```python
from build123d import *

# Parameters (mm, degrees)
F0_W     = 80
F0_H     = 36
F0_W_2   = 74
F0_H_2   = 25
F1_DEPTH = 1.6
F2_DEPTH = 8.5
F3_D     = 2.5
F4_R     = 1


with BuildPart() as f1:
    # F0 (on Top) → F1 (new body)
    with BuildSketch(Plane.XY):
        Rectangle(F0_W, F0_H)
        Rectangle(F0_W_2, F0_H_2, mode=Mode.SUBTRACT)
        Rectangle(F0_W_2, F0_H_2)
    extrude(amount=-F1_DEPTH)

    # F0 (on Top) → F2 (join)
    with BuildSketch(Plane.XY):
        Rectangle(F0_W_2, F0_H_2)
    extrude(amount=F2_DEPTH)

    # F3 (through all)
    with Locations(Plane.XY):
        with Locations((-37.5, 15.5), (37.5, 15.5), (37.5, -15.5), (-37.5, -15.5)):
            Hole(F3_D / 2)

    # F4
    f4_edges = [f1.edges().sort_by_distance(p)[0] for p in [
        (0, 12.5, 8.5),
        (-37, 0, 8.5),
        (0, -12.5, 8.5),
        (37, 0, 8.5),
    ]]
    fillet(f4_edges, radius=F4_R)


solid = f1.part
```
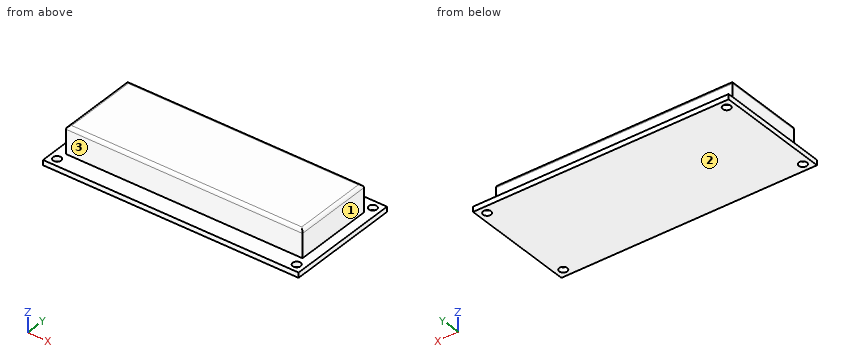
The model under review builds one solid part; all positions refer to its coordinate system, in mm. Face numbers are marked on the shaded views. A direction names the side the tool comes from. Round coordinates to 2 decimals unless told otherwise and drop trailing zeros. Write each loop counter-clockwise with the first axis right and the second up, starting at its lowest first coordinate (ties: lowest second). Pieces come first, ordered by that corner, then holes.
(1) Wall thickness on L1, parallel to Y at x = -37.5, z = -0.4; L2, parallel to Y at x = 27.5, z = 3.5; L3, parallel to X at y = -5.5, z = 1.25: over which ranges is each line inside the solid? List them lowest first.
(2) We need section A-A on y = 15.5. Give the boundary of the cut face in (x, z).
(3) We need section B-B on x = 34. Give the boundary of the cut face in (y, z), and give its area (3 significant figures).
(4) Insertion check: pin 1 (2 mm diameter, centred on y = 2, z = 4.5, fed in from +X); pin 2 (3 mm diameter, centred on x = 11, z = 5, fed in from -Y); pin 3 (3 mm diameter, centred on x = 37.5, y = 15.5, fed in from +Z). Each pin has a flat end and moves straight along its axis. Give the tip position at first contact, or say it passes through.
(5) We need section D-D on z = 6.5. Give the boundary of the cut face in (x, y).
(6) We need section C-C on y = 10. Give the boundary of the cut face in (x, z), and give its area (3 significant figures).
(7) Machinability: for the marked faces 1, 2 and 3, which of the approach directions +Z, -Z, +X, -X, +Y, -Y give a long, thin tool a straight path to every point of the face, cutting with its end or side? Answer none if there is none.
Findings below:
1. L1: y = -18 to -16.75, -14.25 to 14.25, 16.75 to 18
1. L2: y = -12.5 to 12.5
1. L3: x = -37 to 37
2. outline: (-40, -1.6) - (-38.75, -1.6) - (-38.75, 0) - (-40, 0) - close; (-36.25, -1.6) - (36.25, -1.6) - (36.25, 0) - (-36.25, 0) - close; (38.75, -1.6) - (40, -1.6) - (40, 0) - (38.75, 0) - close
3. outline: (-18, -1.6) - (18, -1.6) - (18, 0) - (12.5, 0) - (12.5, 7.5) arc R1 ccw to (11.5, 8.5) - (-11.5, 8.5) arc R1 ccw to (-12.5, 7.5) - (-12.5, 0) - (-18, 0) - close
3. area: 270 mm2
4. pin 1: stops at x = 37
4. pin 2: stops at y = -12.5
4. pin 3: stops at z = 0
5. outline: (-37, -12.5) - (37, -12.5) - (37, 12.5) - (-37, 12.5) - close
6. outline: (-40, -1.6) - (40, -1.6) - (40, 0) - (37, 0) - (37, 7.5) arc R1 ccw to (36, 8.5) - (-36, 8.5) arc R1 ccw to (-37, 7.5) - (-37, 0) - (-40, 0) - close
6. area: 757 mm2
7. face 1: +Z, +X, +Y, -Y
7. face 2: -Z, +X, -X, +Y, -Y
7. face 3: +Z, +X, -X, -Y
